The model under review builds one solid part; all positions refer to its coordinate system, in mm. A direction names the side the tool comes from. Round coordinates to 2 decimals unless told otherwise and drop trailing zeros. Write each loop counter-clockwise with the first axis right and the second up, starting at its lowest first coordinate (ties: lowest second). Pieces come first, ordered by that corner, then holes. Notation, with made-up numbers: (-34.5, 81.25) - (-30.5, 81.25) arc R23 cw to (-30.5, 109.25) - close; hole circle Ø1 at (-21.5, -1). An arc over 180 degrees is marked (long way). Return JSON: item names as keys, results as strings.
from build123d import *
from build123d.topology import SkipClean

# Parameters (mm, degrees)
SKETCH_1_R          = 7.5
EXTRUDE_1_DEPTH     = 10
SKETCH_5_R          = 2.5
CUT_EXTRUDE_1_DEPTH = 14
EXTRUDE_2_DEPTH     = 2
SKETCH_8_R          = 2.5
CUT_EXTRUDE_2_DEPTH = 12


with BuildPart() as part:
    # Sketch 1 → Extrude 1 (new body)
    with BuildSketch(Plane.XY):
        Circle(SKETCH_1_R)
    extrude(amount=EXTRUDE_1_DEPTH)

    # Sketch 4 → Revolve 4 (revolve)
    with SkipClean():  # the faces are left unmerged after this step: merging them gives an invalid solid
        with BuildSketch(Plane(origin=(0, 0, 0), x_dir=(0, -1, 0), z_dir=(-1, 0, 0))):
            with BuildLine():
                Line((-7.5, 10), (7.5, 10))
                ThreePointArc((7.5, 10), (0, 17.5), (-7.5, 10))
            make_face()
        revolve(axis=Axis((0, 7.5, 10), (0, -1, 0)))

    # Sketch 5 → Cut-Extrude 1 (cut)
    with SkipClean():  # the faces are left unmerged after this step: merging them gives an invalid solid
        with BuildSketch(Plane(origin=(0, 0, 0), x_dir=(-1, 0, 0), z_dir=(0, 0, -1))):
            Circle(SKETCH_5_R)
        extrude(amount=-CUT_EXTRUDE_1_DEPTH, mode=Mode.SUBTRACT)

    # Sketch 7 → Extrude 2 (add)
    with BuildSketch(Plane(origin=(0, 0, 5), x_dir=(-1, 0, 0), z_dir=(0, 0, -1))):
        with BuildLine():
            add(Edge.make_bspline(
                [(-27.172583756, 19.274786294), (-14.034416748, 10.081105305), (0, 7.5)],
                knots=[0, 0, 0, 1, 1, 1], degree=2))
            Line((0, 7.5), (27.948278937, 12.158046489))
            ThreePointArc((27.948278937, 12.158046489), (30.006632076, 12.392332685), (32.07817821, 12.412439443))
            Line((32.07817821, 12.412439443), (115.210479882, 8.909799198))
            ThreePointArc((115.210479882, 8.909799198), (118.609182692, 7.374549287), (120, 3.91423134))
            Line((120, 3.91423134), (120, -1.638169923))
            ThreePointArc((120, -1.638169923), (119.541296929, -2.912690922), (118.375596223, -3.602585224))
            Line((118.375596223, -3.602585224), (33.026639247, -19.921306549))
            ThreePointArc((33.026639247, -19.921306549), (30.05093506, -20.03879764), (27.172583756, -19.274786294))
            add(Edge.make_bspline(
                [(27.172583756, -19.274786294), (14.034416748, -10.081105305), (0, -7.5)],
                knots=[0, 0, 0, 1, 1, 1], degree=2))
            Line((0, -7.5), (-27.948278937, -12.158046489))
            ThreePointArc((-27.948278937, -12.158046489), (-30.006632076, -12.392332685), (-32.07817821, -12.412439443))
            Line((-32.07817821, -12.412439443), (-115.210479882, -8.909799198))
            ThreePointArc((-115.210479882, -8.909799198), (-118.609182692, -7.374549287), (-120, -3.91423134))
            Line((-120, -3.91423134), (-120, 1.638169923))
            ThreePointArc((-120, 1.638169923), (-119.541296929, 2.912690922), (-118.375596223, 3.602585224))
            Line((-118.375596223, 3.602585224), (-33.026639247, 19.921306549))
            ThreePointArc((-33.026639247, 19.921306549), (-30.05093506, 20.03879764), (-27.172583756, 19.274786294))
        make_face()
    extrude(amount=-EXTRUDE_2_DEPTH)

    # Sketch 8 → Cut-Extrude 2 (cut)
    with BuildSketch(Plane(origin=(0, 0, 0), x_dir=(-1, 0, 0), z_dir=(0, 0, -1))):
        Circle(SKETCH_8_R)
    extrude(amount=-CUT_EXTRUDE_2_DEPTH, mode=Mode.SUBTRACT)


solid = part.part
(1) Add section C-C (z = 12). Write out the cut boundary in (x, y).
Filled in:
{"outline": "circle Ø14.46 at (0, 0); hole circle Ø5 at (0, 0)"}
(2) Add section A-A (z = 2.5). Write out the cut boundary in (x, y).
Filled in:
{"outline": "circle Ø15 at (0, 0); hole circle Ø5 at (0, 0)"}
(3) For faces 5 (the flat face through (13.8, -9.8, 6)), 6 (the cylindrical face through (-7.493, 0.33, 8.479)), 7 (the cylindrical face through (0.54, -2.44, 6.9)), list the 3-axis set-ups (+Z, -Z, +X, -X, +Y, -Y) from which the entire face can be reached by the end or side of a thin tool; tool diameter is ignored.
Filled in:
{"face 5": "+Z, -Z, -Y", "face 6": "+Z", "face 7": "-Z"}
(4) Mouldability with a two-part tool opening along X and no side actions: class faces 1 (the flat face through (-13.8, 9.8, 6)), 2 (the flat face through (-76.299, -11.648, 5.986)), 3 (the flat face through (59, 0, 7)), 4 (the flat face through (0, 0, 14)) as released by +X, released by -X, zero draft, split by the parting line, or undercut.
Filled in:
{"face 1": "undercut", "face 2": "released by -X", "face 3": "zero draft", "face 4": "undercut"}
(5) Add section D-D (x = -39.5). Write out the cut boundary in (y, z).
Filled in:
{"outline": "(-18.68, 5) - (12.1, 5) - (12.1, 7) - (-18.68, 7) - close"}
(6) Wall thickness on line 1 (Y direction, x = 0, z = 5); line 2 (Z direction, x = 73, y = -2); line 3 (Y direction, x = 0, z = 11): over which ranges is each line inside the solid? List them lowest first.
Filled in:
{"line 1": "y = -7.5 to -2.5, 2.5 to 7.5", "line 2": "z = 5 to 7", "line 3": "y = -7.43 to -2.5, 2.5 to 7.43"}
(7) Add section B-B (x = 103). Write out the cut boundary in (y, z), plus the area to 3 significant figures.
Filled in:
{"outline": "(-9.42, 5) - (6.54, 5) - (6.54, 7) - (-9.42, 7) - close", "area": "31.9 mm2"}
(8) Clearance check with flat-ended pins moving along their axes: pin 1 Ø10 at (x, y) = (78, -2.5) entering from +Z; pin 2 Ø8 at (y, z) = (1, 15.5) entering from +X; pin 3 Ø6 at (x, y) = (-0.5, 0) entering from -Z; pin 4 Ø8 at (x, z) = (20, 5.5) entering from -Y. State where each tip first meets the part, or that it passes through.
Filled in:
{"pin 1": "stops at z = 7", "pin 2": "stops at x = 7.33", "pin 3": "stops at z = 0", "pin 4": "stops at y = -11.5"}
